Autodesk Fusion 360 part; units mm, degrees
sketch "Sketch1" plane through (0, 0, 0) normal (0, 0, 1) x (1, 0, 0)
  circle A0 centre (0, 0) radius 8.5
  dimension "d1" = 17
extrude "Extrude1" add sketch "Sketch1" along normal blind 23
sketch "Sketch2" plane through (0, 0, 23) normal (0, 0, 1) x (-1, 0, 0)
  circle A0 centre (0, 0) radius 8.5
  circle A1 centre (0, 0) radius 3
  dimension "d4" = 6
extrude "Extrude2" add sketch "Sketch2" along normal blind 1 contours A1
sketch "Sketch3" plane through (0, 0, 24) normal (0, 0, 1) x (-1, 0, 0)
  circle A0 centre (0, 0) radius 3
  circle A1 centre (0, 0) radius 1.5
  dimension "d7" = 3
extrude "Extrude3" add sketch "Sketch3" along normal blind 2.5 contours A1
fillet "Fillet1" radius 1 1 edges at (-7.9248, -3.0737, 23)
sketch "Sketch4" plane through (0, 0, 0) normal (0, 0, -1) x (1, 0, 0)
  circle A0 centre (0, 0) radius 8.5
  line L0 (-5, 1.5) -> (-6, 1.5)
  line L1 (-6, 1.5) -> (-6, -1.5)
  line L2 (-6, -1.5) -> (-5, -1.5)
  line L3 (-5, -1.5) -> (-5, 1.5)
  line L4 (-5, 1.5) -> (-6, -1.5) construction
  line L5 (-6, 1.5) -> (-5, -1.5) construction
  line L6 (6, 1.5) -> (5, 1.5)
  line L7 (5, 1.5) -> (5, -1.5)
  line L8 (5, -1.5) -> (6, -1.5)
  line L9 (6, -1.5) -> (6, 1.5)
  line L10 (6, 1.5) -> (5, -1.5) construction
  line L11 (5, 1.5) -> (6, -1.5) construction
  point P0 (-5.5, 0)
  point P1 (5.5, 0)
  dimension "d12" = 1
  dimension "d13" = 1
  dimension "d14" = 3
  dimension "d15" = 3
  dimension "d16" = 5
  dimension "d17" = 5
extrude "Extrude4" add sketch "Sketch4" along normal blind 3.5 contours L0 L1 L2 L3 | L6 L7 L8 L9
sketch "Sketch5" plane through (-6, 0, 0) normal (-1, 0, 0) x (0, -1, 0)
  line L0 (1.5, 0) -> (-1.5, 0)
  line L1 (-1.5, 0) -> (-1.5, -3.5)
  line L2 (-1.5, -3.5) -> (1.5, -3.5)
  line L3 (1.5, -3.5) -> (1.5, 0)
  line L4 (0.25, -2.8) -> (0.25, -0.8)
  arc A0 (0.25, -0.8) -> (-0.25, -0.8) centre (0, -0.8) ccw
  line L5 (-0.25, -0.8) -> (-0.25, -2.8)
  arc A1 (-0.25, -2.8) -> (0.25, -2.8) centre (0, -2.8) ccw
  line L6 (0, -2.8) -> (0, -0.8) construction
  point P0 (0, -1.8)
  dimension "d20" = 2
  dimension "d21" = 0.5
  dimension "d22" = 0.7
extrude "Extrude5" cut sketch "Sketch5" along normal through all contours L4 A0 L5 A1
fillet "Fillet2" radius 1 4 edges at (-5.5, 1.5, -3.5) (-5.5, -1.5, -3.5) (5.5, 1.5, -3.5) (5.5, -1.5, -3.5)
sketch "Sketch6" plane through (0, 0, 26.5) normal (0, 0, 1) x (-1, 0, 0)
  circle A0 centre (0, 0) radius 1.5
  circle A1 centre (0, 0) radius 1.5
  line L0 (0.35, -1.4586) -> (0, -0.8524)
  line L1 (0, -0.8524) -> (-0.35, -1.4586)
  dimension "d26" = 0.7
  dimension "d27" = 0.7
  dimension "d28" = 0.7
extrude "Extrude6" cut sketch "Sketch6" against normal blind 2.5 contours A0 A1 L0 L1 picked at (0.0587, -1.2807)
pattern_circular "C-Pattern1" count 11 over 360 about axis through (0, 0, 24) along (0, 0, 1) of "Extrude6"
Here's how the part is built. I have some questions about the finished solid (model axes, mm). A direction names the side the tool comes from. Coordinates: 2 decimals unless noted, no trailing zeros. Write each loop counter-clockwise with the first axis right and the second up, starting at its lowest first coordinate (ties: lowest second). Pieces come first, ordered by that corner, then holes.
Item 1: I want a section at A-A on z = 23.5. Write out the boundary of the cut face in (x, y).
Item 2: If we mould it in two halves opening along X, with no side actions, what happens to faces 5 (the cylindrical face through (4.57, -7.167, 10.846)), 6 (the flat face through (-5, 0, -2)), 7 (the cylindrical face through (5.507, 1.199, -3.215))? For each: +X half, -X half, draft (parallel to the pull), parting line (faces both ways), or undercut.
Item 3: I want a section at B-B on z = 12.75. Write out the boundary of the cut face in (x, y), and give its area (3 significant figures).
Item 4: If I drill on line 1 (Z direction, x = -3.75, y = 1); line 2 (Z direction, x = -1, y = 0); line 3 (Y direction, x = 1.75, z = 0.5), over which ranges is the centre line in solid material (lowest first)?
Item 5: On a 3-axis mill with a long thin cutter (end or side, diameter ignored), from which of +Z, -Z, +X, -X, +Y, -Y can I reach the whole of each face in a straight line? I mean faces 1 (the flat face through (-5.5, 1.5, -1.2)), 2 (the flat face through (1, -1, 24)), 3 (the flat face through (5, 0, -2)), 4 (the flat face through (5.5, -1.5, -1.2)). Say none if no direction works.
Item 6: Will these pins go through, and if not, where does the flat tip stop? pin 1 (6 mm diameter, centred on x = 6.5, z = 7, fed in from -Y); pin 2 (2.5 mm diameter, centred on y = -0.5, z = -2.5, fed in from -X); pin 3 (1.5 mm diameter, centred on y = 0.5, z = -2.5, fed in from +X).
Findings below:
1. outline: circle Ø6 at (0, 0)
2. face 5: parting line
2. face 6: undercut
2. face 7: draft
3. outline: circle Ø17 at (0, 0)
3. area: 227 mm2
4. line 1: z = 0 to 23
4. line 2: z = 0 to 26.5
4. line 3: y = -8.32 to 8.32
5. face 1: -Z, +X, -X, +Y
5. face 2: +Z
5. face 3: -Z, +Y, -Y
5. face 4: -Z, +X, -X, -Y
6. pin 1: stops at y = -7.75
6. pin 2: stops at x = -6
6. pin 3: stops at x = 6
